Part model, mm, in its own coordinate system. A direction names the side the tool comes from. Coordinates: 2 decimals unless noted, no trailing zeros. Loops run counter-clockwise (first coordinate to the right, second up) from the corner with the lowest first, then second, coordinate; pieces in that order, holes last.
```python
from build123d import *

# Parameters (mm, degrees)
RESSALTO_EXTRUS_O1_DEPTH = 3
RESSALTO_EXTRUS_O2_DEPTH = 11
CORTE_EXTRUS_O1_DEPTH    = 6
ESBO_O3_R                = 2
CORTE_EXTRUS_O2_DEPTH    = 23.2
FILETE1_R                = 1
FILETE2_R                = 2
CORTE_EXTRUS_O3_DEPTH    = 3


with BuildPart() as part:
    # Esboço1 → Ressalto-extrusão1 (new body)
    with BuildSketch(Plane.XY):
        with BuildLine():
            Line((-10, 12.5), (10, 12.5))
            ThreePointArc((10, 12.5), (22.5, 0), (10, -12.5))
            Line((10, -12.5), (-10, -12.5))
            ThreePointArc((-10, -12.5), (-22.5, 0), (-10, 12.5))
        make_face()
        with BuildLine():
            Line((-10, 9.7), (10, 9.7))
            ThreePointArc((10, 9.7), (19.7, 0), (10, -9.7))
            Line((10, -9.7), (-10, -9.7))
            ThreePointArc((-10, -9.7), (-19.7, 0), (-10, 9.7))
        make_face(mode=Mode.SUBTRACT)
    extrude(amount=RESSALTO_EXTRUS_O1_DEPTH)

    # Esboço1<2> → Ressalto-extrusão2 (add)
    with BuildSketch(Plane.XY):
        with BuildLine():
            Line((-10, 9.7), (10, 9.7))
            ThreePointArc((10, 9.7), (19.7, 0), (10, -9.7))
            Line((10, -9.7), (-10, -9.7))
            ThreePointArc((-10, -9.7), (-19.7, 0), (-10, 9.7))
        make_face()
    extrude(amount=RESSALTO_EXTRUS_O2_DEPTH)

    # Esboço2 → Corte-extrusão1 (cut)
    with BuildSketch(Plane.XY.offset(11)):
        with BuildLine():
            Line((-10, -9.7), (-4, -9.7))
            Line((-4, -9.7), (-4, -6.7))
            Line((-4, -6.7), (4, -6.7))
            Line((4, -6.7), (4, -9.7))
            Line((4, -9.7), (10, -9.7))
            ThreePointArc((10, -9.7), (19.7, 0), (10, 9.7))
            Line((10, 9.7), (4, 9.7))
            Line((4, 9.7), (4, 6.7))
            Line((4, 6.7), (-4, 6.7))
            Line((-4, 6.7), (-4, 9.7))
            Line((-4, 9.7), (-10, 9.7))
            ThreePointArc((-10, 9.7), (-19.7, 0), (-10, -9.7))
        make_face()
    extrude(amount=-CORTE_EXTRUS_O1_DEPTH, mode=Mode.SUBTRACT)

    # Esboço3 → Corte-extrusão2 (cut, through all)
    with BuildSketch(Plane.XZ.offset(9.7)):
        with Locations((0, 8)):
            Circle(ESBO_O3_R)
    extrude(amount=-CORTE_EXTRUS_O2_DEPTH, mode=Mode.SUBTRACT)

    # Filete1
    filete1_edges = [part.edges().sort_by_distance(p)[0] for p in [
        (-4, 6.7, 8),
        (4, 6.7, 8),
        (4, -6.7, 8),
        (-4, -6.7, 8),
        (-4, -8.2, 11),
        (4, -8.2, 11),
        (4, 8.2, 11),
        (-4, 8.2, 11),
    ]]
    fillet(filete1_edges, radius=FILETE1_R)

    # Filete2
    filete2_edges = [part.edges().sort_by_distance(p)[0] for p in [
        (0, 12.5, 0),
        (22.5, 0, 0),
        (0, -12.5, 0),
        (-22.5, 0, 0),
    ]]
    fillet(filete2_edges, radius=FILETE2_R)

    # Esboço4 → Corte-extrusão3 (cut)
    with BuildSketch(Plane.XY.offset(5)):
        with BuildLine():
            Line((-10, -8.7), (-4, -8.7))
            Line((-4, -8.7), (-4, -7.7))
            ThreePointArc((-4, -7.7), (-3.707106781, -6.992893219), (-3, -6.7))
            Line((-3, -6.7), (3, -6.7))
            ThreePointArc((3, -6.7), (3.707106781, -6.992893219), (4, -7.7))
            Line((4, -7.7), (4, -8.7))
            Line((4, -8.7), (10, -8.7))
            ThreePointArc((10, -8.7), (18.7, 0), (10, 8.7))
            Line((10, 8.7), (4, 8.7))
            Line((4, 8.7), (4, 7.7))
            ThreePointArc((4, 7.7), (3.707106781, 6.992893219), (3, 6.7))
            Line((3, 6.7), (-3, 6.7))
            ThreePointArc((-3, 6.7), (-3.707106781, 6.992893219), (-4, 7.7))
            Line((-4, 7.7), (-4, 8.7))
            Line((-4, 8.7), (-10, 8.7))
            ThreePointArc((-10, 8.7), (-18.7, 0), (-10, -8.7))
        make_face()
    extrude(amount=-CORTE_EXTRUS_O3_DEPTH, mode=Mode.SUBTRACT)


solid = part.part
```
Q1. Saw through at B-B (z = 3.75). List the corners of the cut face in (x, y).
Q2. Drop flat-ended pins along their axis: P1, Ø0.6, axis at y = 8.5, z = 6, coming from the -X side; P2, Ø1, axis at y = -8.5, z = 5, coming from the +X side; P3, Ø8.5, axis at x = -8, y = -1, coming from the +Z side. Give the stop position or say it passes through.
Q3. Probe line 1 (Z direction, x = 0, y = 8.8); line 2 (Y direction, x = -8, z = 4); line 3 (Z direction, x = 17, y = 4.5). List the from-to ranges inside material, lowest first.
Q4. Saw through at D-D (x = -7.5). List the corners of the cut face in (y, z).
Q5. Saw through at C-C (y = 0). List the corners of the cut face in (x, z).
Q6. Mould opens along X. For faces 4 (the flat face through (-4, -9, 7)), 5 (the flat face through (19, 0, 5)), 6 (the cylindrical face through (18.698, -0.191, 3.521)), 7 (the cylindrical face through (-3.715, 8.221, 10.699)) say: released by +X, released by -X, zero draft, split by the parting line, or undercut.
Q7. Tool access for faces 1 (the cylindrical face through (-19.698, -0.213, 3.986)), 2 (the cylindrical face through (19.698, 0.213, 3.986)), 3 (the cylindrical face through (-18.698, 0.191, 3.521)): list every direction of +Z, -Z, +X, -X, +Y, -Y with a clear straight run to the whole face (end or side of a thin tool).
Q8. Saw through at A-A (x = 0). List the corners of the cut face in (y, z), plus the area to 3 significant figures.
Checked values:
1. outline: (-10, -9.7) - (10, -9.7) arc R9.7 ccw to (10, 9.7) - (-10, 9.7) arc R9.7 ccw to start; hole (-10, -8.7) - (-4, -8.7) - (-4, -7.7) arc R1 cw to (-3, -6.7) - (3, -6.7) arc R1 cw to (4, -7.7) - (4, -8.7) - (10, -8.7) arc R8.7 ccw to (10, 8.7) - (4, 8.7) - (4, 7.7) arc R1 cw to (3, 6.7) - (-3, 6.7) arc R1 cw to (-4, 7.7) - (-4, 8.7) - (-10, 8.7) arc R8.7 ccw to start
2. P1: stops at x = -4
2. P2: stops at x = 15.49
2. P3: stops at z = 2
3. line 1: z = 0 to 6, 10 to 11
3. line 2: y = -9.7 to -8.7, 8.7 to 9.7
3. line 3: z = 0 to 2
4. outline: (-12.5, 2) arc R2 ccw to (-10.5, 0) - (10.5, 0) arc R2 ccw to (12.5, 2) - (12.5, 3) - (9.7, 3) - (9.7, 5) - (8.7, 5) - (8.7, 2) - (-8.7, 2) - (-8.7, 5) - (-9.7, 5) - (-9.7, 3) - (-12.5, 3) - close
5. outline: (-22.5, 2) arc R2 ccw to (-20.5, 0) - (20.5, 0) arc R2 ccw to (22.5, 2) - (22.5, 3) - (19.7, 3) - (19.7, 5) - (18.7, 5) - (18.7, 2) - (-18.7, 2) - (-18.7, 5) - (-19.7, 5) - (-19.7, 3) - (-22.5, 3) - close
6. face 4: undercut
6. face 5: zero draft
6. face 6: undercut
6. face 7: released by -X
7. face 1: +Z, -X
7. face 2: +Z, +X
7. face 3: +Z
8. outline: (-12.5, 2) arc R2 ccw to (-10.5, 0) - (10.5, 0) arc R2 ccw to (12.5, 2) - (12.5, 3) - (9.7, 3) - (9.7, 6) - (6.7, 6) - (6.7, 2) - (-6.7, 2) - (-6.7, 6) - (-9.7, 6) - (-9.7, 3) - (-12.5, 3) - close; (-9.7, 10) - (-6.7, 10) - (-6.7, 11) - (-9.7, 11) - close; (6.7, 10) - (9.7, 10) - (9.7, 11) - (6.7, 11) - close
8. area: 83.9 mm2
